Model file for the job. Use its own axes, mm. Face numbers are marked on the shaded views. A direction names the side the tool comes from. Coordinates: 2 decimals unless noted, no trailing zeros. Order: outer loops, then holes, each group sorted by start corner. A loop starts at its lowest first (then second) coordinate and runs counter-clockwise, first axis right, second up. Notation, with made-up numbers: (-18.75, -31.75) -> (8.25, -31.75) arc R19 ccw to (8.25, -8.75) -> close; hole circle Ø3 at (84.25, -29.5). An arc over 180 degrees is marked (long way). Use CSV: the item, a comma, the result in double quotes. Start each with the question number.
(1) Cut at A-A on z = 12. Write the cut outline in (x, y), plus the area to 3 significant figures.
(2) Pin check, flat tips, straight feed: pin 1 Ø6 at (x, y) = (-4, 1.5) entering from -Z; pin 2 Ø6 at (x, z) = (-9, -5.5) entering from -Y; pin 3 Ø5.5 at (x, z) = (8, -11.5) entering from +Y; pin 4 Ø5 at (y, z) = (5, 11.5) entering from -X. Stop position of each tip, or through.
(3) Cut at D-D on x = -9.75. Write the cut outline in (y, z).
(4) Probe L1, parallel to Z at x = 2, y = 9.5; L2, parallel to Z at x = 6.75, y = 6; L3, parallel to Y at x = 9.5, z = 14. List the from-to ranges inside material, lowest first.
(5) Cut at C-C on y = 3. Give the number of separate pieces and of enclosed holes in the cut face, plus the area to 3 significant figures.
(6) Tool access for the marked faces 1, 2 and 3: list every direction of +Z, -Z, +X, -X, +Y, -Y with a clear straight run to the whole face (end or side of a thin tool).
Autodesk Inventor part; units mm, degrees
ref_plane "YZ Plane" through (0, 0, 0) normal (1, 0, 0) x (0, 1, 0)
ref_plane "XZ Plane" through (0, 0, 0) normal (0, 1, 0) x (-1, 0, 0)
ref_plane "XY Plane" through (0, 0, 0) normal (0, 0, 1) x (1, 0, 0)
sketch "Sketch1" plane through (0, 0, 0) normal (0, 1, 0) x (-1, 0, 0)
  line L0 (0, 0) -> (28.575, 0)
  line L1 (28.575, 0) -> (0, 0)
  line L2 (0, 0) -> (-14.2875, -24.7467)
  line L3 (0, 0) -> (28.575, 0) construction
  line L4 (0, 0) -> (-14.2875, 24.7467)
  line L5 (0, 0) -> (28.575, 0) construction
  circle A0 centre (28.575, 0) radius 2.54
  circle A1 centre (-14.2875, -24.7467) radius 2.54
  circle A2 centre (-14.2875, 24.7467) radius 2.54
  circle A3 centre (0, 0) radius 3.175
  circle A4 centre (0, 0) radius 6.35
  line L6 (-1.5875, -2.7496) -> (0, 0)
  line L7 (0, 0) -> (-6.35, 0)
  circle A5 centre (-14.2875, 24.7467) radius 3.81
  circle A6 centre (28.575, 0) radius 3.81
  circle A7 centre (-14.2875, -24.7467) radius 3.81
  line L8 (30.6811, 3.175) -> (-12.1814, 27.9217)
  line L9 (28.2054, -3.792) -> (-10.8187, -26.3226)
  line L10 (-18.0975, 24.7467) -> (-18.0975, -24.7467)
  line L11 (0, 0) -> (5.0525, -8.8146)
  line L12 (0, 0) -> (5.1463, 8.7602)
  line L13 (0, 0) -> (-10.16, 0)
  arc A8 (28.2054, -3.792) -> (-10.8187, -26.3226) centre (24.4473, -42.344) ccw
  arc A9 (-10.8187, 26.3226) -> (28.2054, 3.792) centre (24.4473, 42.344) ccw
  arc A10 (-17.3867, -22.5305) -> (-17.3867, 22.5305) centre (-48.8947, 0) ccw
  point P0 (5.1074, 8.7829)
  point P1 (-10.16, 0.0317)
  point P2 (30.2716, 3.4114)
  point P3 (28.2054, 3.792)
  point P4 (-10.8187, 26.3226)
  point P5 (-17.3867, 22.5305)
  point P6 (-17.3867, -22.5305)
  dimension "d9" = 6.35
  dimension "d41" = 12.7
  dimension "d0" = 28.575
  dimension "d1" = 28.575
  dimension "d2" = 120
  dimension "d3" = 28.575
  dimension "d4" = 120
  dimension "d5" = 5.08
  dimension "d6" = 5.08
  dimension "d7" = 5.08
  dimension "d42" = 7.62
  dimension "d43" = 7.62
  dimension "d44" = 7.62
  dimension "d47" = 10.16
  dimension "d48" = 10.16
  dimension "d49" = 10.16
  dimension "d52" = 360
extrude "Extrusion4" add sketch "Sketch1" along normal blind 12.7 contours A3 L12 A4 L0 | L0 A4 L11 A3 | A3 L11 A4 L2 | L2 A4 L7 A3 | A3 L7 A4 L4 | L4 A4 L12 A3 | A4 L12 A9 A6 L0 | L0 A6 A8 L11 A4 | A4 L11 A8 A7 L2 | L2 A7 A10 L13 A4 | A4 L13 A10 A5 L4 | L4 A5 A9 L12 A4 | A6 L8 | A7 | A5 picked at (31.8987, 0.5122)
sketch "Sketch19" plane through (0, 12.7, 0) normal (0, 1, 0) x (1, 0, 0)
  arc A0 (17.3867, 22.5305) -> (10.8187, 26.3226) centre (14.2875, 24.7467) ccw
  line L0 (5.3975, 9.3487) -> (0.1191, 12.3962)
  arc A1 (-28.2054, 3.792) -> (10.8187, 26.3226) centre (-24.4473, 42.344) ccw
  arc A2 (-28.2054, 3.792) -> (-30.6811, -3.175) centre (-28.575, 0) ccw
  line L1 (-30.6811, -3.175) -> (-30.2716, -3.4114)
  arc A3 (-30.2716, -3.4114) -> (-28.2054, -3.792) centre (-28.575, 0) ccw
  arc A4 (10.8187, -26.3226) -> (-28.2054, -3.792) centre (-24.4473, -42.344) ccw
  arc A5 (10.8187, -26.3226) -> (17.3867, -22.5305) centre (14.2875, -24.7467) ccw
  arc A6 (17.3867, 22.5305) -> (17.3867, -22.5305) centre (48.8947, 0) ccw
  arc A7 (17.3867, 22.5305) -> (10.8187, 26.3226) centre (14.2875, 24.7467) ccw
  circle A8 centre (-28.575, 0) radius 2.54
  circle A9 centre (0, 0) radius 3.175
  circle A10 centre (14.2875, -24.7467) radius 2.54
  circle A11 centre (14.2875, 24.7467) radius 2.54
  line L2 (10.6759, 6.3013) -> (5.3975, 9.3487)
  arc A12 (-28.2054, 3.792) -> (10.8187, 26.3226) centre (-24.4473, 42.344) ccw
  point P0 (17.3867, 22.5305)
  point P1 (10.8187, 26.3226)
  point P2 (0.1191, 12.3962)
extrude "Extrusion9" cut sketch "Sketch19" against normal blind 6.35 contours A6 L2 L0 A1 A0
sketch "Sketch20" plane through (0, 6.35, 0) normal (0, 1, 0) x (1, 0, 0)
  line L0 (0, 0) -> (5.3975, 9.3487)
  line L1 (10.6759, 6.3013) -> (0.1191, 12.3962)
  line L2 (5.3975, 9.3487) -> (8.5725, 14.848)
  line L3 (8.5725, 14.848) -> (5.3975, 16.6811)
  line L4 (5.3975, 16.6811) -> (8.5725, 14.848)
  arc A0 (17.3867, 22.5305) -> (17.3867, -22.5305) centre (48.8947, 0) ccw
  line L5 (12.2997, 12.6961) -> (8.5725, 14.848)
  arc A1 (0.1191, 12.3962) -> (10.8187, 26.3226) centre (-24.4473, 42.344) ccw
  arc A2 (17.3867, 22.5305) -> (10.8187, 26.3226) centre (14.2875, 24.7467) ccw
  line L6 (8.5725, 14.848) -> (4.3283, 17.2984)
  point P0 (4.8453, 16.9999)
  dimension "d113" = 6.35
extrude "Extrusion10" cut sketch "Sketch20" against normal blind 6.35 contours L5 L3 L6 A1 A2 A0
pattern_circular "Circular Pattern2" count 3 over 360 about axis through (0, 0, 0) along (0, 1, 0) of "Extrusion9", "Extrusion10"
sketch "Sketch21" plane through (0, 12.7, 0) normal (0, 1, 0) x (1, 0, 0)
  point P0 (0, 0)
sketch "Sketch22" plane through (0, 6.35, 0) normal (0, 1, 0) x (1, 0, 0)
  line L0 (0, 0) -> (8.5725, 14.848)
  line L1 (4.8453, 16.9999) -> (12.2997, 12.6961)
  line L2 (10.6759, 6.3013) -> (0.1191, 12.3962)
  line L3 (5.3975, 9.3487) -> (8.5725, 14.848)
  line L4 (5.3975, 9.3487) -> (6.985, 12.0984)
  arc A0 (0.1191, 12.3962) -> (4.8453, 16.9999) centre (-24.4473, 42.344) ccw
  line L5 (2.6088, 14.625) -> (6.985, 12.0984)
  line L6 (6.985, 12.0984) -> (11.3612, 9.5718)
  arc A1 (12.2997, 12.6961) -> (12.2997, -12.6961) centre (48.8947, 0) ccw
hole "Hole8" at (6.985, 6.35, -12.0984) direction (0, -1, 0) diameter 2.1129 depth 7.7978
pattern_circular "Circular Pattern3" count 3 over 360 about axis through (0, 0, 0) along (0, 1, 0) of "Hole8"
properties part number "stability copy"
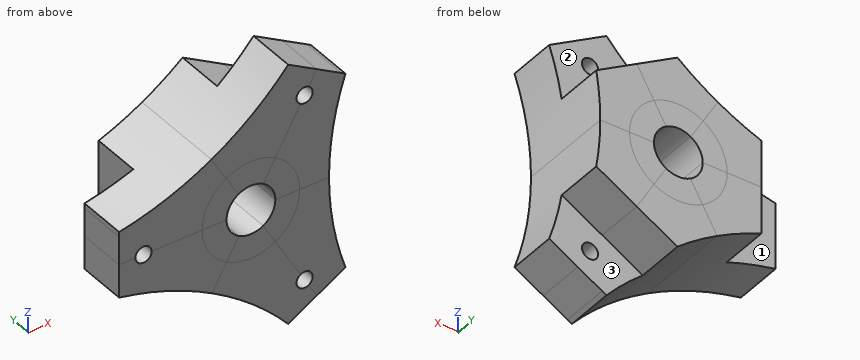
Outcome:
1,outline,"(-0.37, 0) -> (5.93, 0) -> (5.93, 6.35) -> (0.81, 6.35) -> (0.81, 12.7) -> (-0.37, 12.7) -> close; (8.04, 0) -> (12.07, 0) -> (12.07, 6.35) -> (8.04, 6.35) -> close"
1,area,"73.1 mm2"
2,pin 1,"z = -11.51"
2,pin 2,"y = 0"
2,pin 3,"y = 6.35"
2,pin 4,"x = -4.74"
3,outline,"(0, -6.51) -> (12.7, -6.51) -> (12.7, 6.51) -> (0, 6.51) -> close"
4,L1,"-11.31 to -2.47, 2.47 to 11.31"
4,L2,"-15.9 to -13.13, -11.07 to 11.07, 13.13 to 15.9"
4,L3,"0 to 6.35"
5,separate pieces,"1"
5,enclosed holes,"4"
5,area,"538 mm2"
6,face 1,"+Z, -Z, -X, +Y"
6,face 2,"+Z, +X, +Y"
6,face 3,"-Z, +X, +Y"
